Build history of the part. All positions in model axes, mm. Round coordinates to 2 decimals unless told otherwise and drop trailing zeros. Order: outer loops, then holes, each group sorted by start corner. A loop starts at its lowest first (then second) coordinate and runs counter-clockwise, first axis right, second up. Notation, with made-up numbers: (-33, 65) -> (-10, 65) arc R22 ccw to (-10, 87) -> close; hole circle Ø5 at (64, -16). An arc over 180 degrees is marked (long way). Write item = value, one per line.
from build123d import *

# Parameters (mm, degrees)
CYLINDER_R     = 1.1
CYLINDER_DEPTH = 10
BOX008_W       = 7
BOX008_H       = 7
BOX008_DEPTH   = 4.5


with BuildPart() as hole:
    # Cylinder → Cylinder (new body)
    with BuildSketch(Plane.XY):
        Circle(CYLINDER_R)
    extrude(amount=CYLINDER_DEPTH)


with BuildPart() as stand_hole_cut:
    # Box008 → Box008 (new body)
    with BuildSketch(Plane(origin=(-3.5, -3.5, 0), x_dir=(1, 0, 0), z_dir=(0, 0, 1))):
        with Locations((3.5, 3.5)):
            Rectangle(BOX008_W, BOX008_H)
    extrude(amount=BOX008_DEPTH)

    # Cut003002: cut hole
    add(hole.part, mode=Mode.SUBTRACT)


solid = stand_hole_cut.part
Q1. Mould opens along X. For faces 1 (the face through (1.05, 0.33, 2.22)), 2 (the face through (-1, 1, 4.5)), 3 (the face through (-3.5, 0, 2)), 4 (the face through (3.5, 0, 2)) say: released by +X, released by -X, zero draft, split by the parting line, or undercut.
Check values:
face_1 = undercut
face_2 = zero draft
face_3 = released by -X
face_4 = released by +X
Q2. Cut at C-C, the plane z = 3.65. List the corners of the cut face in (x, y), and give its area (3 significant figures).
Check values:
outline = (-3.5, -3.5) -> (3.5, -3.5) -> (3.5, 3.5) -> (-3.5, 3.5) -> close; hole circle Ø2.2 at (0, 0)
area = 45.2 mm²
Q3. Probe probe 1 along X at (y, z) = (0, 3.5); probe 2 along Y at (x, z) = (-1, 1.4). List the from-to ranges inside material, lowest first.
Check values:
probe_1 = -3.5 to -1.1, 1.1 to 3.5
probe_2 = -3.5 to -0.46, 0.46 to 3.5
Q4. Cut at A-A, the plane x = 0. List the corners of the cut face in (y, z).
Check values:
outline = (-3.5, 0) -> (-1.1, 0) -> (-1.1, 4.5) -> (-3.5, 4.5) -> close; (1.1, 0) -> (3.5, 0) -> (3.5, 4.5) -> (1.1, 4.5) -> close
